```python
from build123d import *

# Parameters (mm, degrees)
SKETCH1_W           = 3
SKETCH1_H           = 3
SKETCH1_H_2         = 10
SKETCH1_W_2         = 244
BOSS_EXTRUDE1_DEPTH = 3
SKETCH1_4_W         = 3
SKETCH1_4_H         = 3
SKETCH1_4_H_2       = 10
SKETCH1_4_W_2       = 244
BOSS_EXTRUDE2_DEPTH = 75
FILLET1_R           = 5
FILLET2_R           = 5


with BuildPart() as part:
    # Sketch1 → Boss-Extrude1 (new body)
    with BuildSketch(Plane.XY):
        with Locations((-80.354290742, 77.454120293)):
            Rectangle(SKETCH1_W, SKETCH1_H)
        with Locations((-80.354290742, 70.954120293)):
            Rectangle(SKETCH1_W, SKETCH1_H_2)
        with Locations((-80.354290742, 64.454120293)):
            Rectangle(SKETCH1_W, SKETCH1_H)
        with Locations((-80.354290742, 57.954120293)):
            Rectangle(SKETCH1_W, SKETCH1_H_2)
        with Locations((-80.354290742, 51.454120293)):
            Rectangle(SKETCH1_W, SKETCH1_H)
        with Locations((-80.354290742, 44.954120293)):
            Rectangle(SKETCH1_W, SKETCH1_H_2)
        with Locations((-80.354290742, 38.454120293)):
            Rectangle(SKETCH1_W, SKETCH1_H)
        with Locations((-80.354290742, 31.954120293)):
            Rectangle(SKETCH1_W, SKETCH1_H_2)
        with Locations((-80.354290742, 25.454120293)):
            Rectangle(SKETCH1_W, SKETCH1_H)
        with Locations((43.145709258, 25.454120293)):
            Rectangle(SKETCH1_W_2, SKETCH1_H)
        with Locations((43.145709258, 31.954120293)):
            Rectangle(SKETCH1_W_2, SKETCH1_H_2)
        with Locations((43.145709258, 38.454120293)):
            Rectangle(SKETCH1_W_2, SKETCH1_H)
        with Locations((43.145709258, 44.954120293)):
            Rectangle(SKETCH1_W_2, SKETCH1_H_2)
        with Locations((43.145709258, 51.454120293)):
            Rectangle(SKETCH1_W_2, SKETCH1_H)
        with Locations((43.145709258, 57.954120293)):
            Rectangle(SKETCH1_W_2, SKETCH1_H_2)
        with Locations((43.145709258, 64.454120293)):
            Rectangle(SKETCH1_W_2, SKETCH1_H)
        with Locations((43.145709258, 70.954120293)):
            Rectangle(SKETCH1_W_2, SKETCH1_H_2)
        with Locations((43.145709258, 77.454120293)):
            Rectangle(SKETCH1_W_2, SKETCH1_H)
        with Locations((166.645709258, 77.454120293)):
            Rectangle(SKETCH1_W, SKETCH1_H)
        with Locations((166.645709258, 70.954120293)):
            Rectangle(SKETCH1_W, SKETCH1_H_2)
        with Locations((166.645709258, 64.454120293)):
            Rectangle(SKETCH1_W, SKETCH1_H)
        with Locations((166.645709258, 57.954120293)):
            Rectangle(SKETCH1_W, SKETCH1_H_2)
        with Locations((166.645709258, 51.454120293)):
            Rectangle(SKETCH1_W, SKETCH1_H)
        with Locations((166.645709258, 44.954120293)):
            Rectangle(SKETCH1_W, SKETCH1_H_2)
        with Locations((166.645709258, 38.454120293)):
            Rectangle(SKETCH1_W, SKETCH1_H)
        with Locations((166.645709258, 31.954120293)):
            Rectangle(SKETCH1_W, SKETCH1_H_2)
        with Locations((166.645709258, 25.454120293)):
            Rectangle(SKETCH1_W, SKETCH1_H)
    extrude(amount=BOSS_EXTRUDE1_DEPTH)

    # Sketch1<4> → Boss-Extrude2 (add)
    with BuildSketch(Plane.XY):
        with Locations((-80.354290742, 77.454120293)):
            Rectangle(SKETCH1_4_W, SKETCH1_4_H)
        with Locations((-80.354290742, 70.954120293)):
            Rectangle(SKETCH1_4_W, SKETCH1_4_H_2)
        with Locations((-80.354290742, 64.454120293)):
            Rectangle(SKETCH1_4_W, SKETCH1_4_H)
        with Locations((-80.354290742, 57.954120293)):
            Rectangle(SKETCH1_4_W, SKETCH1_4_H_2)
        with Locations((-80.354290742, 51.454120293)):
            Rectangle(SKETCH1_4_W, SKETCH1_4_H)
        with Locations((-80.354290742, 44.954120293)):
            Rectangle(SKETCH1_4_W, SKETCH1_4_H_2)
        with Locations((43.145709258, 51.454120293)):
            Rectangle(SKETCH1_4_W_2, SKETCH1_4_H)
        with Locations((43.145709258, 64.454120293)):
            Rectangle(SKETCH1_4_W_2, SKETCH1_4_H)
        with Locations((43.145709258, 77.454120293)):
            Rectangle(SKETCH1_4_W_2, SKETCH1_4_H)
        with Locations((-80.354290742, 38.454120293)):
            Rectangle(SKETCH1_4_W, SKETCH1_4_H)
        with Locations((-80.354290742, 31.954120293)):
            Rectangle(SKETCH1_4_W, SKETCH1_4_H_2)
        with Locations((-80.354290742, 25.454120293)):
            Rectangle(SKETCH1_4_W, SKETCH1_4_H)
        with Locations((43.145709258, 25.454120293)):
            Rectangle(SKETCH1_4_W_2, SKETCH1_4_H)
        with Locations((43.145709258, 38.454120293)):
            Rectangle(SKETCH1_4_W_2, SKETCH1_4_H)
        with Locations((166.645709258, 77.454120293)):
            Rectangle(SKETCH1_4_W, SKETCH1_4_H)
        with Locations((166.645709258, 70.954120293)):
            Rectangle(SKETCH1_4_W, SKETCH1_4_H_2)
        with Locations((166.645709258, 64.454120293)):
            Rectangle(SKETCH1_4_W, SKETCH1_4_H)
        with Locations((166.645709258, 57.954120293)):
            Rectangle(SKETCH1_4_W, SKETCH1_4_H_2)
        with Locations((166.645709258, 51.454120293)):
            Rectangle(SKETCH1_4_W, SKETCH1_4_H)
        with Locations((166.645709258, 44.954120293)):
            Rectangle(SKETCH1_4_W, SKETCH1_4_H_2)
        with Locations((166.645709258, 38.454120293)):
            Rectangle(SKETCH1_4_W, SKETCH1_4_H)
        with Locations((166.645709258, 31.954120293)):
            Rectangle(SKETCH1_4_W, SKETCH1_4_H_2)
        with Locations((166.645709258, 25.454120293)):
            Rectangle(SKETCH1_4_W, SKETCH1_4_H)
    extrude(amount=BOSS_EXTRUDE2_DEPTH)

    # Fillet1
    fillet1_edges = [part.edges().sort_by_distance(p)[0] for p in [
        (-81.854290742, 78.954120293, 37.5),
        (168.145709258, 78.954120293, 37.5),
    ]]
    fillet(fillet1_edges, radius=FILLET1_R)

    # Fillet2
    # the kernel refuses this fillet: 5 mm, written as the material it takes off along each edge
    with BuildSketch(Plane(origin=(168.145709258, 73.954120293, 75), x_dir=(-1, 0, 0), z_dir=(0, -1, 0)), Plane(origin=(-81.854290742, 11.454120293, 75), x_dir=(1, 0, 0), z_dir=(0, 1, 0))) as fillet2_piece_1:
        with BuildLine():
            CenterArc((FILLET2_R, FILLET2_R), FILLET2_R, 180, 90)
            Line((0, FILLET2_R), (0, 0))
            Line((0, 0), (FILLET2_R, 0))
        make_face()
    extrude(amount=62.5, mode=Mode.SUBTRACT)
    with BuildSketch(Plane(origin=(-76.854290742, 73.954120293, 75), x_dir=(0, 1, 0), z_dir=(1, 0, 0))) as fillet2_piece_2:
        with BuildLine():
            CenterArc((5 - FILLET2_R, -FILLET2_R), FILLET2_R, 0, 90)
            Line((5 - FILLET2_R, 0), (5, 0))
            Line((5, 0), (5, -FILLET2_R))
        make_face()
    revolve(axis=Axis((-76.854290742, 73.954120293, 75), (0, 0, 1)), revolution_arc=90, mode=Mode.SUBTRACT)
    with BuildSketch(Plane(origin=(-76.854290742, 78.954120293, 75), x_dir=(0, 0, -1), z_dir=(1, 0, 0))) as fillet2_piece_3:
        with BuildLine():
            CenterArc((FILLET2_R, -FILLET2_R), FILLET2_R, 90, 90)
            Line((0, -FILLET2_R), (0, 0))
            Line((0, 0), (FILLET2_R, 0))
        make_face()
    extrude(amount=240, mode=Mode.SUBTRACT)
    with BuildSketch(Plane(origin=(163.145709258, 73.954120293, 75), x_dir=(0, 1, 0), z_dir=(-1, 0, 0))) as fillet2_piece_4:
        with BuildLine():
            CenterArc((5 - FILLET2_R, FILLET2_R), FILLET2_R, 270, 90)
            Line((5 - FILLET2_R, 0), (5, 0))
            Line((5, 0), (5, FILLET2_R))
        make_face()
    revolve(axis=Axis((163.145709258, 73.954120293, 75), (0, 0, -1)), revolution_arc=90, mode=Mode.SUBTRACT)


solid = part.part
```
Part model, mm, in its own coordinate system. A direction names the side the tool comes from. Give positions to 0.01 mm unless a question says otherwise; leave off trailing zeros. Order: outer loops, then holes, each group sorted by start corner. A loop starts at its lowest first (then second) coordinate and runs counter-clockwise, first axis right, second up. Notation, with made-up numbers: M 48,85.5 L 88,85.5 A17 cw 88,111.5 Z; hole C -16,26.25 d11. An arc over 180 degrees is marked long. Use a Markdown table: item, result. Add a question column.
(1) 3-axis set-ups, long thin cutter, end or side, ignore diameter. For faces 4 (the face through (41, 65.954, 38)), 5 (the face through (-80.43, 77.45, 34.51)): which of +Z, -Z, +X, -X, +Y, -Y reach the whole face in a straight line?
(2) Saw through at B-B, the plane y = 43. Give the cut face in (x, z).
(3) Saw through at C-C, the plane x = 93.5. Give the cut face in (y, z), and give its area (3 significant figures).
(4) Drop flat-ended pins along their axis: P1, Ø5, axis at x = 87.5, y = 59, coming from the +Z side; P2, Ø8, axis at x = 99.5, y = 73, coming from the +Z side. Give the stop position or say it passes through.
(5) Saw through at A-A, the plane z = 19. Give the cut face in (x, y).
(6) Probe line 1 along Y through (x, z) = (34, 56); line 2 along X through (y, z) = (70.5, 50); line 3 along Y through (x, z) = (138.5, 71). List the from-to ranges inside material, lowest first. Write a range as [from, to].
(7) Mould opens along Y. For faces 1 (the face through (41, 23.954, 37)), 2 (the face through (41, 52, 0)), 3 (the face through (41, 32, 3)) say: +Y half, -Y half, draft (parallel to the pull), parting line (faces both ways), or undercut.
Answer key:
| question | item | result |
|---|---|---|
| 1 | face 4 | +Z |
| 1 | face 5 | +Z, -Z, -X, +Y |
| 2 | outline | M -81.85,0 L 168.15,0 L 168.15,70 A5 ccw 165.15,74.58 L 165.15,3 L -78.85,3 L -78.85,74.58 A5 ccw -81.85,70 Z |
| 3 | outline | M 23.95,0 L 78.95,0 L 78.95,70 A5 ccw 75.95,74.58 L 75.95,3 L 65.95,3 L 65.95,75 L 62.95,75 L 62.95,3 L 52.95,3 L 52.95,75 L 49.95,75 L 49.95,3 L 39.95,3 L 39.95,75 L 36.95,75 L 36.95,3 L 26.95,3 L 26.95,75 L 23.95,75 Z |
| 3 | area | 1,240 mm^2 |
| 4 | P1 | z = 3 |
| 4 | P2 | z = 74.58 |
| 5 | outline | M -81.85,23.95 L 168.15,23.95 L 168.15,73.95 A5 ccw 163.15,78.95 L -76.85,78.95 A5 ccw -81.85,73.95 Z; hole M -78.85,26.95 L 165.15,26.95 L 165.15,36.95 L -78.85,36.95 Z; hole M -78.85,39.95 L 165.15,39.95 L 165.15,49.95 L -78.85,49.95 Z; hole M -78.85,52.95 L 165.15,52.95 L 165.15,62.95 L -78.85,62.95 Z; hole M -78.85,65.95 L 165.15,65.95 L 165.15,75.95 L -78.85,75.95 Z |
| 6 | line 1 | [23.95, 26.95], [36.95, 39.95], [49.95, 52.95], [62.95, 65.95], [75.95, 78.95] |
| 6 | line 2 | [-81.85, -78.85], [165.15, 168.15] |
| 6 | line 3 | [23.95, 26.95], [36.95, 39.95], [49.95, 52.95], [62.95, 65.95], [75.95, 78.85] |
| 7 | face 1 | -Y half |
| 7 | face 2 | draft |
| 7 | face 3 | undercut |
